```python
from build123d import *

# Parameters (mm, degrees)
F0_W     = 117.3992
F0_H     = 31.391128
F1_DEPTH = 5
F2_R     = 2
F3_R     = 2
F4_R     = 2
F5_R     = 2


with BuildPart() as f1:
    # F0 (on Top) → F1 (new body)
    with BuildSketch(Plane.XY):
        Rectangle(F0_W, F0_H)
    extrude(amount=F1_DEPTH)

    # F2
    f2_edges = [f1.edges().sort_by_distance(p)[0] for p in [
        (0, -15.695564, 5),
    ]]
    fillet(f2_edges, radius=F2_R)

    # F3
    f3_edges = [f1.edges().sort_by_distance(p)[0] for p in [
        (58.6996, 1, 5),
        (0, 15.695564, 5),
    ]]
    fillet(f3_edges, radius=F3_R)

    # F4
    f4_edges = [f1.edges().sort_by_distance(p)[0] for p in [
        (-58.6996, 0, 5),
    ]]
    fillet(f4_edges, radius=F4_R)

    # F5
    f5_edges = [f1.edges().sort_by_distance(p)[0] for p in [
        (-58.6996, 0, 0),
        (0, -15.695564, 0),
        (1, 15.695564, 0),
        (58.6996, 1, 0),
    ]]
    fillet(f5_edges, radius=F5_R)


solid = f1.part
```
Here's how the part is built. I have some questions about the finished solid (model axes, mm). Coordinates: 2 decimals unless noted, no trailing zeros. Write each loop counter-clockwise with the first axis right and the second up, starting at its lowest first coordinate (ties: lowest second). Pieces come first, ordered by that corner, then holes. Notation, with made-up numbers: M 74.5,-21 L 81.5,-21 A27 cw 81.5,17 Z; hole C -19.5,49.25 d10. An arc over 180 degrees is marked long. Answer as CSV lines item,"result". Start each with the question number.
Q1. Suppose I cut it at A-A, the plane x = -32.5. List the corners of the cut face in (y, z) for me, then the cut area to 3 significant figures.
Q2. Suppose I cut it at B-B, the plane z = 0.95. List the corners of the cut face in (x, y) for me, then the cut area to 3 significant figures.
Q3. I need wall thicknesses on probe 1 along X at (y, z) = (11.5, 1.7); probe 2 along X at (y, z) = (8, 3.95); probe 3 along Y at (x, z) = (-23, 1). Which ranges of each line are inside material? Lowest first, please. Write a range as [from, to].
Entries:
1,outline,"M -15.7,2 A2 ccw -13.7,0 L 13.7,0 A2 ccw 15.7,2 L 15.7,3 A2 ccw 13.7,5 L -13.7,5 A2 ccw -15.7,3 Z"
1,area,"154 mm²"
2,outline,"M -58.4,-13.7 A1.7 ccw -56.7,-15.4 L 56.7,-15.4 A1.7 ccw 58.4,-13.7 L 58.4,15.4 L -56.7,15.4 A1.7 ccw -58.4,13.7 Z"
2,area,"3,600 mm²"
3,probe 1,"x = [-58.68, 58.68]"
3,probe 2,"x = [-58.46, 58.46]"
3,probe 3,"y = [-15.43, 15.43]"
